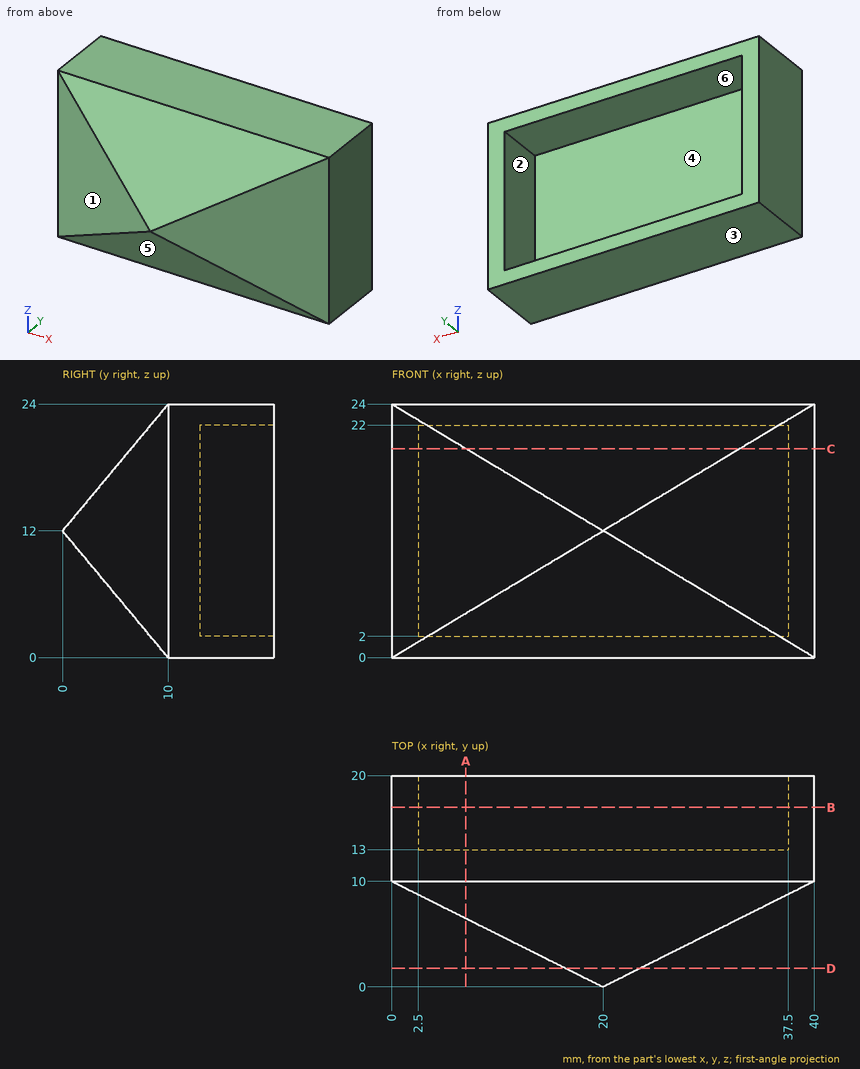
Geometry check sheet. Reference: drawing and pictorial views, mm from the part's lowest x, y, z. A direction names the side the tool comes from. Round coordinates to 2 decimals unless told otherwise and drop trailing zeros. Loops run counter-clockwise (first coordinate to the right, second up) from the corner with the lowest first, then second, coordinate; pieces in that order, holes last.
1. Mould release check, pull along X, two halves, no side actions. Record for the marked faces 1, 2, 3 and 4: released by +X, released by -X, zero draft, split by the parting line, or undercut.
2. Sectioned sample at C-C on z = 19.75. Record the boundary of the cut face in (x, y), and give its area (3 significant figures).
3. Sectioned sample at D-D on y = 1.75. Record the boundary of the cut face in (x, z).
4. Gauge pin test, flat ends, axial feed: pin 1 Ø1 at (x, z) = (17, 6.5) entering from +Y; pin 2 Ø6 at (x, z) = (29.5, 17) entering from -Y; pin 3 Ø12 at (x, z) = (33, 15.5) entering from -Y. Record the tip position at first contact, or that the pin passes through.
5. Scan lines: probe 1 along X at (y, z) = (18.25, 19.5); probe 2 along Z at (x, y) = (33, 15.5); probe 3 along Y at (x, z) = (35, 6). Record each from-to range of solid material in increasing order.
6. Sectioned sample at B-B on y = 17. Record the boundary of the cut face in (x, z).
7. Sectioned sample at A-A on x = 7. Record the boundary of the cut face in (y, z), and give its area (3 significant figures).
8. Set-up check for the marked faces 5 and 6: record each of +Z, -Z, +X, -X, +Y, -Y from which the full face is reachable in a straight line by a thin tool's end or side.
Recorded:
1. face 1: released by -X
1. face 2: undercut
1. face 3: zero draft
1. face 4: undercut
2. outline: (0, 10) - (7.08, 6.46) - (32.92, 6.46) - (40, 10) - (40, 20) - (37.5, 20) - (37.5, 13) - (2.5, 13) - (2.5, 20) - (0, 20) - close
2. area: 272 mm2
3. outline: (16.5, 9.9) - (23.5, 9.9) - (23.5, 14.1) - (16.5, 14.1) - close
4. pin 1: stops at y = 13
4. pin 2: stops at y = 3.34
4. pin 3: stops at y = 3.5
5. probe 1: x = 0 to 2.5, 37.5 to 40
5. probe 2: z = 0 to 2, 22 to 24
5. probe 3: y = 7.5 to 13
6. outline: (0, 0) - (40, 0) - (40, 24) - (0, 24) - close; hole (2.5, 2) - (37.5, 2) - (37.5, 22) - (2.5, 22) - close
7. outline: (6.5, 4.2) - (10, 0) - (20, 0) - (20, 2) - (13, 2) - (13, 22) - (20, 22) - (20, 24) - (10, 24) - (6.5, 19.8) - close
7. area: 169 mm2
8. face 5: -Z, +X, -X, -Y
8. face 6: +Y
